```python
from build123d import *

# Parameters (mm, degrees)
SKETCH_R     = 1.6
PAD_DEPTH    = 3
PAD001_DEPTH = 20
SKETCH002_W  = 9.48
SKETCH002_H  = 9.48
POCKET_DEPTH = 1.56
CHAMFER_SIZE = 8
FILLET_R     = 3


with BuildPart() as part:
    # Sketch → Pad (new body)
    with BuildSketch(Plane.XY):
        Polygon((-10, 10), (10, 10), (10, -10), (-10, -10), (-25, -10), (-25, 10), align=None)
        Circle(SKETCH_R, mode=Mode.SUBTRACT)
        with BuildLine():
            ThreePointArc((-20.9, 1.6), (-22.5, 0), (-20.9, -1.6))
            Line((-20.9, -1.6), (-11.6, -1.6))
            ThreePointArc((-11.6, -1.6), (-10, 0), (-11.6, 1.6))
            Line((-11.6, 1.6), (-20.9, 1.6))
        make_face(mode=Mode.SUBTRACT)
    extrude(amount=PAD_DEPTH)

    # Sketch001 (on Face3 of Pad) → Pad001 (join)
    with BuildSketch(Plane.XZ.offset(10)):
        Polygon((-4.74, 3), (4.74, 3), (2.94, 4.56), (-2.94, 4.56), align=None)
    extrude(amount=-PAD001_DEPTH)

    # Sketch002 (on Face18 of Pad001) → Pocket (cut)
    with BuildSketch(Plane.XY.offset(4.56)):
        Rectangle(SKETCH002_W, SKETCH002_H)
    extrude(amount=-POCKET_DEPTH, mode=Mode.SUBTRACT)

    # Chamfer
    chamfer_edges = [part.edges().sort_by_distance(p)[0] for p in [
        (-25, 10, 1.5),
        (-25, -10, 1.5),
    ]]
    chamfer(chamfer_edges, length=CHAMFER_SIZE)

    # Fillet
    fillet_edges = [part.edges().sort_by_distance(p)[0] for p in [
        (10, 10, 1.5),
        (10, -10, 1.5),
    ]]
    fillet(fillet_edges, radius=FILLET_R)


solid = part.part
```
Can you work these out from the model? Positions are in its coordinate system, mm. A direction names the side the tool comes from. Round coordinates to 2 decimals unless told otherwise and drop trailing zeros. Loops run counter-clockwise (first coordinate to the right, second up) from the corner with the lowest first, then second, coordinate; pieces in that order, holes last.
Item 1: Suppose I cut it at C-C, the plane z = 1.35. Write out the boundary of the cut face in (x, y).
Item 2: Suppose I cut it at A-A, the plane y = 0. Write out the boundary of the cut face in (x, z), then the cut area to 3 significant figures.
Item 3: If we mould it in two halves opening along Y, with no side actions, what happens to faces 1 (the flat face through (-16, 1.6, 1)), 2 (the cylindrical face through (9.1, 9.14, 1.52)), 3 (the flat face through (-5, -10, 2)), 4 (the flat face through (-3.83, 7.33, 3.79))? For each: +Y half, -Y half, draft (parallel to the pull), parting line (faces both ways), or undercut.
Item 4: Please list where these lines run through material, in increasing order: L1, parallel to Y at x = 0, z = 2.35; L2, parallel to X at y = 0.75, z = 1.7; L3, parallel to Y at x = 2, z = 3.45.
Item 5: Suppose I cut it at D-D, the plane y = -5.5. Write out the boundary of the cut face in (x, z), then the cut area to 3 significant figures.
Item 6: Suppose I cut it at B-B, the plane x = 0. Write out the boundary of the cut face in (y, z).
Item 7: Which directions (+Z, -Z, +X, -X, +Y, -Y) give clear straight access to the entire face, cutting with the end or side of a thin tool? Please do faces 5 (the flat face through (-5, 10, 2)), 6 (the flat face through (-16, -1.6, 1)), 7 (the flat face through (0, 4.74, 4)).
Item 8: Will these pins go through, and if not, where does the flat tip stop? pin 1 Ø4 at (x, y) = (-12.5, 1) entering from -Z; pin 2 Ø2 at (x, y) = (-17, -2.5) entering from +Z.
Reported:
1. outline: (-25, -2) - (-17, -10) - (7, -10) arc R3 ccw to (10, -7) - (10, 7) arc R3 ccw to (7, 10) - (-17, 10) - (-25, 2) - close; hole (-20.9, -1.6) - (-11.6, -1.6) arc R1.6 ccw to (-11.6, 1.6) - (-20.9, 1.6) arc R1.6 ccw to start; hole circle Ø3.2 at (0, 0)
2. outline: (-25, 0) - (-22.5, 0) - (-22.5, 3) - (-25, 3) - close; (-10, 0) - (-1.6, 0) - (-1.6, 3) - (-10, 3) - close; (1.6, 0) - (10, 0) - (10, 3) - (1.6, 3) - close
2. area: 57.9 mm2
3. face 1: undercut
3. face 2: +Y half
3. face 3: -Y half
3. face 4: draft
4. L1: y = -10 to -1.6, 1.6 to 10
4. L2: x = -25 to -22.31, -10.19 to -1.41, 1.41 to 10
4. L3: y = -10 to -4.74, 4.74 to 10
5. outline: (-21.5, 0) - (10, 0) - (10, 3) - (4.74, 3) - (2.94, 4.56) - (-2.94, 4.56) - (-4.74, 3) - (-21.5, 3) - close
5. area: 106 mm2
6. outline: (-10, 0) - (-1.6, 0) - (-1.6, 3) - (-4.74, 3) - (-4.74, 4.56) - (-10, 4.56) - close; (1.6, 0) - (10, 0) - (10, 4.56) - (4.74, 4.56) - (4.74, 3) - (1.6, 3) - close
7. face 5: +Z, -Z, +X, -X, +Y
7. face 6: +Z, -Z
7. face 7: +Z, +X, -X
8. pin 1: stops at z = 0
8. pin 2: stops at z = 3
